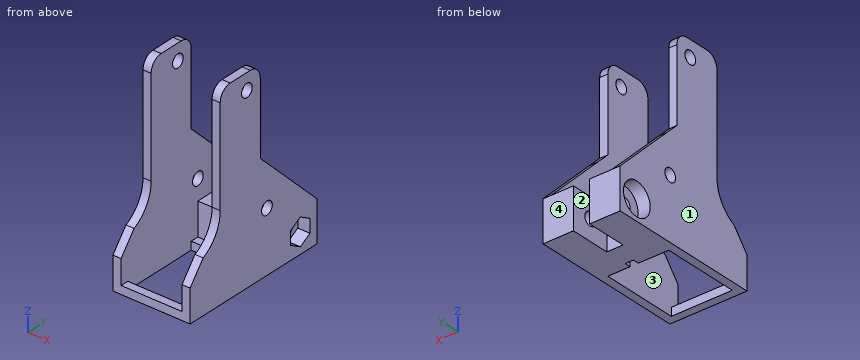
```python
from build123d import *

# Parameters (mm, degrees)
SKETCH001_W          = 17.4
SKETCH001_H          = 38
PAD001_DEPTH         = 2
SKETCH002_R          = 1.6
PAD_DEPTH            = 2
SKETCH005_R          = 1.6
PAD002_DEPTH         = 2
PAD003_DEPTH         = 10
SKETCH006_W          = 4
SKETCH006_H          = 10
POCKET001_DEPTH      = 0.001
POCKET001_DEPTH_BACK = 48.001
SKETCH007_R          = 1.6
POCKET_DEPTH         = 9.501
POCKET_DEPTH_BACK    = 9.501
SKETCH008_R          = 4
POCKET002_DEPTH      = 3
POCKET003_DEPTH      = 3
SKETCH004_R          = 1.6
POCKET004_DEPTH      = 9.501
POCKET004_DEPTH_BACK = 9.501
CHAMFER_SIZE         = 13.99
CHAMFER001_SIZE      = 3
FILLET_R             = 8.99
CHAMFER002_SIZE      = 4
FILLET001_R          = 3


with BuildPart() as part:
    # Sketch001 → Pad001 (new body)
    with BuildSketch(Plane.XY):
        with Locations((0, -19)):
            Rectangle(SKETCH001_W, SKETCH001_H)
        Polygon((7.5, -17), (7.5, -36), (-7.5, -36), (-7.5, -17), (0, -17), (0, -15.5), (2, -15.5), (2, -17), align=None, mode=Mode.SUBTRACT)
    extrude(amount=PAD001_DEPTH)

    # Sketch002 (on DatumPlane) → Pad (join)
    with BuildSketch(Plane.YZ.offset(-9.5)):
        Polygon((0, 24), (0, 0), (-38, 0), (-38, 12), (-29, 12), (-29, 48), (-17, 48), (-17, 24), align=None)
        with Locations((-21, 44)):
            Circle(SKETCH002_R, mode=Mode.SUBTRACT)
    extrude(amount=PAD_DEPTH)

    # Sketch005 (on DatumPlane) → Pad002 (join)
    with BuildSketch(Plane.YZ.offset(9.5)):
        Polygon((0, 24), (0, 0), (-38, 0), (-38, 12), (-29, 12), (-29, 48), (-17, 48), (-17, 24), align=None)
        with Locations((-21, 44)):
            Circle(SKETCH005_R, mode=Mode.SUBTRACT)
    extrude(amount=-PAD002_DEPTH)

    # Sketch → Pad003 (join)
    with BuildSketch(Plane.XY):
        Polygon((-2, 0), (-8.7, 0), (-8.7, -15), (8.7, -15), (8.7, 0), (2, 0), (2, -10), (-2, -10), align=None)
    extrude(amount=PAD003_DEPTH)

    # Sketch006 → Pocket001 (cut, two sides)
    with BuildSketch(Plane.XY) as pocket001_sk:
        with Locations((0, -5)):
            Rectangle(SKETCH006_W, SKETCH006_H)
    extrude(amount=-POCKET001_DEPTH, mode=Mode.SUBTRACT)
    extrude(pocket001_sk.sketch, amount=POCKET001_DEPTH_BACK, mode=Mode.SUBTRACT)

    # Sketch007 → Pocket (cut, two sides)
    with BuildSketch(Plane.YZ) as pocket_sk:
        with Locations((-5, 5)):
            Circle(SKETCH007_R)
    extrude(amount=-POCKET_DEPTH, mode=Mode.SUBTRACT)
    extrude(pocket_sk.sketch, amount=POCKET_DEPTH_BACK, mode=Mode.SUBTRACT)

    # Sketch008 (on DatumPlane) → Pocket002 (cut)
    with BuildSketch(Plane.YZ.offset(-9.5)):
        with Locations((-5, 5)):
            Circle(SKETCH008_R)
    extrude(amount=POCKET002_DEPTH, mode=Mode.SUBTRACT)

    # Sketch009 (on DatumPlane) → Pocket003 (cut)
    with BuildSketch(Plane.YZ.offset(9.5)):
        Polygon((-2.125, 3.340118), (-2.125, 6.659882), (-5, 8.319764), (-7.875, 6.659882), (-7.875, 3.340118), (-5, 1.680236), align=None)
    extrude(amount=-POCKET003_DEPTH, mode=Mode.SUBTRACT)

    # Sketch004 → Pocket004 (cut, two sides)
    with BuildSketch(Plane.YZ) as pocket004_sk:
        with Locations((-15, 15)):
            Circle(SKETCH004_R)
    extrude(amount=-POCKET004_DEPTH, mode=Mode.SUBTRACT)
    extrude(pocket004_sk.sketch, amount=POCKET004_DEPTH_BACK, mode=Mode.SUBTRACT)

    # Chamfer
    chamfer_edges = [part.edges().sort_by_distance(p)[0] for p in [
        (-8.5, 0, 24),
        (8.5, 0, 24),
    ]]
    chamfer(chamfer_edges, length=CHAMFER_SIZE)

    # Chamfer001
    chamfer001_edges = [part.edges().sort_by_distance(p)[0] for p in [
        (8.5, -17, 24),
        (-8.5, -17, 24),
    ]]
    chamfer(chamfer001_edges, length=CHAMFER001_SIZE)

    # Fillet
    fillet_edges = [part.edges().sort_by_distance(p)[0] for p in [
        (-8.5, -29, 12),
        (8.5, -29, 12),
    ]]
    fillet(fillet_edges, radius=FILLET_R)

    # Chamfer002
    chamfer002_edges = [part.edges().sort_by_distance(p)[0] for p in [
        (-8.5, -38, 12),
        (8.5, -38, 12),
    ]]
    chamfer(chamfer002_edges, length=CHAMFER002_SIZE)

    # Fillet001
    fillet001_edges = [part.edges().sort_by_distance(p)[0] for p in [
        (-8.5, -29, 48),
        (8.5, -29, 48),
        (8.5, -17, 48),
        (-8.5, -17, 48),
    ]]
    fillet(fillet001_edges, radius=FILLET001_R)


solid = part.part
```
Read the model definition and answer for the solid it produces. Units are mm, in the model's axes. Face numbers are marked on the shaded views. Coordinates: 2 decimals unless noted, no trailing zeros. Order: outer loops, then holes, each group sorted by start corner. A loop starts at its lowest first (then second) coordinate and runs counter-clockwise, first axis right, second up. Notation, with made-up numbers: (-16.5, 59.25) - (-1.5, 59.25) arc R17 cw to (-1.5, 92.25) - close; hole circle Ø6 at (76.25, 12.25). An arc over 180 degrees is marked (long way). Answer as a JSON object with one key per item and string values. Group by question number.
Item 1: Flat-ended cylindrical pins translate along their axes: P1, Ø5, axis at y = -5, z = 5, coming from the +X side; P2, Ø6, axis at x = -2.5, z = 27, coming from the +Y side; P3, Ø8, axis at y = -6.5, z = 6, coming from the -X side; P4, Ø2, axis at x = -3.5, y = -15.5, coming from the +Z side. Find the tip coordinate at first contact, or state that the pin passes through.
Item 2: The mould has two halves that part along X. Classify the marked faces 1, 2, 3 and 4: +X half, -X half, draft (parallel to the pull), parting line (faces both ways), or undercut.
Item 3: Section C-C (z = 44) is taken. Give the vertices of the cut face in (x, y).
Item 4: Section A-A (z = 5) is taken. Give the vertices of the cut face in (x, y) (3 decimals), plus the area to 3 significant figures.
Item 5: Section B-B (y = -21) is taken. Give the vertices of the cut face in (x, z).
Item 6: Consider probe 1 along Z at (x, y) = (5.4, -5); probe 2 along X at (y, z) = (-33, 9); probe 3 along Z at (x, y) = (-8.8, -15). Determine where each line is inside the solid, lowest interval first. Write a range as from..to.
Item 7: Section D-D (y = -31.5) is taken. Give the vertices of the cut face in (x, z).
Results are:
{
 "1": {"P1": "stops at x = 6.5", "P2": "passes through", "P3": "stops at x = -9.5", "P4": "stops at z = 10"},
 "2": {"face 1": "-X half", "face 2": "undercut", "face 3": "undercut", "face 4": "draft"},
 "3": {"outline": "(-9.5, -29) - (-7.5, -29) - (-7.5, -22.6) - (-9.5, -22.6) - close; (-9.5, -19.4) - (-7.5, -19.4) - (-7.5, -17) - (-9.5, -17) - close; (7.5, -29) - (9.5, -29) - (9.5, -22.6) - (7.5, -22.6) - close; (7.5, -19.4) - (9.5, -19.4) - (9.5, -17) - (7.5, -17) - close"},
 "4": {"outline": "(-9.5, -38) - (-7.5, -38) - (-7.5, -15) - (7.5, -15) - (7.5, -38) - (9.5, -38) - (9.5, -7.875) - (6.5, -7.875) - (6.5, -6.6) - (2, -6.6) - (2, -10) - (-2, -10) - (-2, -6.6) - (-6.5, -6.6) - (-6.5, -9) - (-9.5, -9) - close; (-9.5, -1) - (-6.5, -1) - (-6.5, -3.4) - (-2, -3.4) - (-2, 0) - (-9.5, 0) - close; (2, -3.4) - (6.5, -3.4) - (6.5, -2.125) - (9.5, -2.125) - (9.5, 0) - (2, 0) - close", "area": "267 mm^2"},
 "5": {"outline": "(-9.5, 0) - (-7.5, 0) - (-7.5, 42.4) - (-9.5, 42.4) - close; (-9.5, 45.6) - (-7.5, 45.6) - (-7.5, 48) - (-9.5, 48) - close; (7.5, 0) - (9.5, 0) - (9.5, 42.4) - (7.5, 42.4) - close; (7.5, 45.6) - (9.5, 45.6) - (9.5, 48) - (7.5, 48) - close"},
 "6": {"probe 1": "z = 0..3.4, 6.6..10", "probe 2": "x = -9.5..-7.5, 7.5..9.5", "probe 3": "z = 0..13.4, 16.6..25"},
 "7": {"outline": "(-9.5, 0) - (-7.5, 0) - (-7.5, 14.77) - (-9.5, 14.77) - close; (7.5, 0) - (9.5, 0) - (9.5, 14.77) - (7.5, 14.77) - close"}
}
